Design review of the part built by this model. Coordinates are the model's own, in mm. A direction names the side the tool comes from. Coordinates: 2 decimals unless noted, no trailing zeros. Loops run counter-clockwise (first coordinate to the right, second up) from the corner with the lowest first, then second, coordinate; pieces in that order, holes last. Notation, with made-up numbers: M -29,22.25 L 19,22.25 A37 cw 19,61.25 Z; hole C -19.75,-34 d8. An arc over 180 degrees is marked long. One line per item, written item: value.
Autodesk Inventor part; units mm, degrees
ref_plane "YZ Plane" through (0, 0, 0) normal (1, 0, 0) x (0, 1, 0)
ref_plane "XZ Plane" through (0, 0, 0) normal (0, 1, 0) x (-1, 0, 0)
ref_plane "XY Plane" through (0, 0, 0) normal (0, 0, 1) x (1, 0, 0)
sketch "Sketch1" plane through (0, 0, 0) normal (0, 1, 0) x (-1, 0, 0)
  line L0 (9.525, 9.525) -> (-9.525, 9.525)
  line L1 (-9.525, 9.525) -> (-9.525, -9.525)
  line L2 (-9.525, -9.525) -> (9.525, -9.525)
  line L3 (9.525, -9.525) -> (9.525, 9.525)
  point P0 (0, 0)
  dimension "d0" = 19.05
  dimension "d1" = 19.05
  dimension "d2" = 9.525
  dimension "d3" = 9.525
extrude "Extrusion1" add sketch "Sketch1" along normal blind 19.05
sketch "Sketch2" plane through (0, 0, 0) normal (0, -1, 0) x (1, 0, 0)
  line L0 (6.35, 6.35) -> (-6.35, 6.35)
  line L1 (-6.35, 6.35) -> (-6.35, -6.35)
  line L2 (-6.35, -6.35) -> (6.35, -6.35)
  line L3 (6.35, -6.35) -> (6.35, 6.35)
  point P0 (0, 0)
  dimension "d6" = 12.7
  dimension "d7" = 12.7
  dimension "d8" = 6.35
  dimension "d9" = 6.35
extrude "Extrusion2" cut sketch "Sketch2" against normal blind 12.7
sketch "Sketch3" plane through (0, 19.05, 0) normal (0, 1, 0) x (1, 0, 0)
  circle A0 centre (0, 0) radius 4.826
  circle A1 centre (0, 0) radius 2.159
  dimension "d12" = 9.652
  dimension "d13" = 4.318
extrude "Extrusion3" cut sketch "Sketch3" against normal blind 0.889
sketch "Sketch4" plane through (0, 19.05, 0) normal (0, 1, 0) x (1, 0, 0)
  circle A0 centre (0, 0) radius 0.3619
  dimension "d16" = 0.7239
extrude "Extrusion4" cut sketch "Sketch4" against normal through all
sketch "Sketch5" plane through (0, 18.161, 0) normal (0, 1, 0) x (1, 0, 0)
  circle A0 centre (3.4925, 0) radius 1.3335
  circle A1 centre (0, 0) radius 2.159
  line L0 (0, 0) -> (3.4925, 0) construction
  dimension "d19" = 2.667
  dimension "d20" = 3.4925
extrude "Extrusion5" cut sketch "Sketch5" against normal through all contours A0
sketch "Sketch7" plane through (-9.525, 0, 9.525) normal (0, 0, 1) x (1, 0, 0)
  line L0 (0, 0) -> (0, 19.05)
  line L1 (0, 12.7) -> (19.05, 12.7)
  line L2 (19.05, 12.7) -> (19.05, 0)
  line L3 (19.05, 0) -> (0, 0)
  line L4 (0, 0) -> (0, 12.7)
  point P0 (9.525, 0)
  dimension "d23" = 12.7
  dimension "d24" = 19.05
extrude "Extrusion6" cut sketch "Sketch7" against normal through all
fillet "Fillet1" radius 3.175 4 edges at (-9.525, 15.875, 9.525) (9.525, 15.875, 9.525) (9.525, 15.875, -9.525) (-9.525, 15.875, -9.525)
properties part number "Unit_v1"
(1) Tool access review of faces 4 (the cylindrical face through (-0.28, 18.61, -2.14)), 5 (the flat face through (0, 12.7, -2)): name each direction out of +Z, -Z, +X, -X, +Y, -Y from which nothing blocks a thin tool from reaching the whole face with its end or side.
Reply:
face 4: +Y
face 5: +Z, -Z, +X, -X, -Y
(2) We need section D-D on z = -1.75. State the section outline as (x, y) points (3 decimals), then the cut area to 3 significant figures.
Reply:
outline: M -9.525,12.7 L 9.525,12.7 L 9.525,19.05 L 4.498,19.05 L 4.498,18.161 L 1.264,18.161 L 1.264,19.05 L -1.264,19.05 L -1.264,18.161 L -4.498,18.161 L -4.498,19.05 L -9.525,19.05 Z
area: 115 mm2
(3) We need section A-A on x = 0. State the section outline as (y, z) points (3 decimals), then the cut area to 3 significant figures.
Reply:
outline: M 12.7,-9.525 L 19.05,-9.525 L 19.05,-4.826 L 18.161,-4.826 L 18.161,-2.159 L 19.05,-2.159 L 19.05,-0.362 L 12.7,-0.362 Z; M 12.7,0.362 L 19.05,0.362 L 19.05,2.159 L 18.161,2.159 L 18.161,4.826 L 19.05,4.826 L 19.05,9.525 L 12.7,9.525 Z
area: 112 mm2
(4) To check wall thickness, follow line 1 along X through (y, z) = (17.05, 0) (3 decimals); line 2 along X through (y, z) = (18.6, 0) (3 decimals); line 3 along X through (y, z) = (13.75, -0.25) (3 decimals). State the ranges of each line that lie inside material, in increasing order. Write a range as [from, to].
Reply:
line 1: x = [-9.525, -0.362], [0.362, 2.159], [4.826, 9.525]
line 2: x = [-9.525, -4.826], [-2.159, -0.362], [0.362, 2.159], [4.826, 9.525]
line 3: x = [-9.525, -0.262], [0.262, 2.183], [4.802, 9.525]
(5) We need section B-B on y = 14. State how many separate pieces and enclosed holes the cut face has, then the cut area to 3 significant figures.
Reply:
separate pieces: 1
enclosed holes: 2
area: 348 mm2
(6) Mouldability with a two-part tool opening along Z and no side actions: class faces 1 (the cylindrical face through (8.57, 15.92, 8.62)), 2 (the flat face through (-2.2, 18.161, 1)), 3 (the flat face through (-9.525, 16, 0)) as released by +Z, released by -Z, zero draft, split by the parting line, or undercut.
Reply:
face 1: released by +Z
face 2: undercut
face 3: zero draft
(7) We need section C-C on x = -4. State the section outline as (y, z) points (3 decimals), then the cut area to 3 significant figures.
Reply:
outline: M 12.7,-9.525 L 19.05,-9.525 L 19.05,-2.7 L 18.161,-2.7 L 18.161,2.7 L 19.05,2.7 L 19.05,9.525 L 12.7,9.525 Z
area: 116 mm2
(8) Insertion check: pin 1 (3 mm diameter, centred on y = 13.5, z = -7, fed in from +X) (3 decimals). The pin has a flat end and moves straight along its axis. Give the tip position at first contact, or say it passes through.
Reply:
pin 1: stops at x = 9.525
